Answer from the drawing. Dimensions are ordinates in mm from the lowest x, y and z of the part. A direction names the side the tool comes from. Coordinates: 2 decimals unless noted, no trailing zeros. Write each loop counter-clockwise with the first axis right and the second up, starting at its lowest first coordinate (ties: lowest second). Pieces come first, ordered by that corner, then holes.
(1) Section B-B on y = 19 is taken. Write down the section's boundary in (x, z).
(2) Section C-C on x = 40 is taken. Write down the section's boundary in (y, z), then the cut area to 3 significant figures.
(3) Section A-A on z = 28.5 is taken. Write down the section's boundary in (x, y), then the cut area to 3 significant figures.
(4) Section D-D on z = 3.5 is taken. Write down the section's boundary in (x, y).
(5) Find the intervals of material crossed by probe 1 along X at (y, z) = (90.5, 7.5); probe 2 along Y at (x, z) = (20, 24.5); probe 3 along Y at (x, z) = (23, 16), in increasing order.
(6) The mould has two halves that part along X. Classify the marked faces 4, 5 and 6: +X half, -X half, draft (parallel to the pull), parting line (faces both ways), or undercut.
(7) Given pin 1 (16 mm diameter, centred on y = 10, z = 12.5, fed in from +X); pin 2 (10 mm diameter, centred on y = 21, z = 10, fed in from -X); pin 3 (3 mm diameter, centred on x = 28.5, z = 6, fed in from +Y), each flat-ended and moving along its own axis, determine where each tip first touches the part or whether it passes through.
(8) Which of the six approach directions +Z, -Z, +X, -X, +Y, -Y give full straight-line access (tool end or side, diameter ignored) to the marked faces 1, 2 and 3?
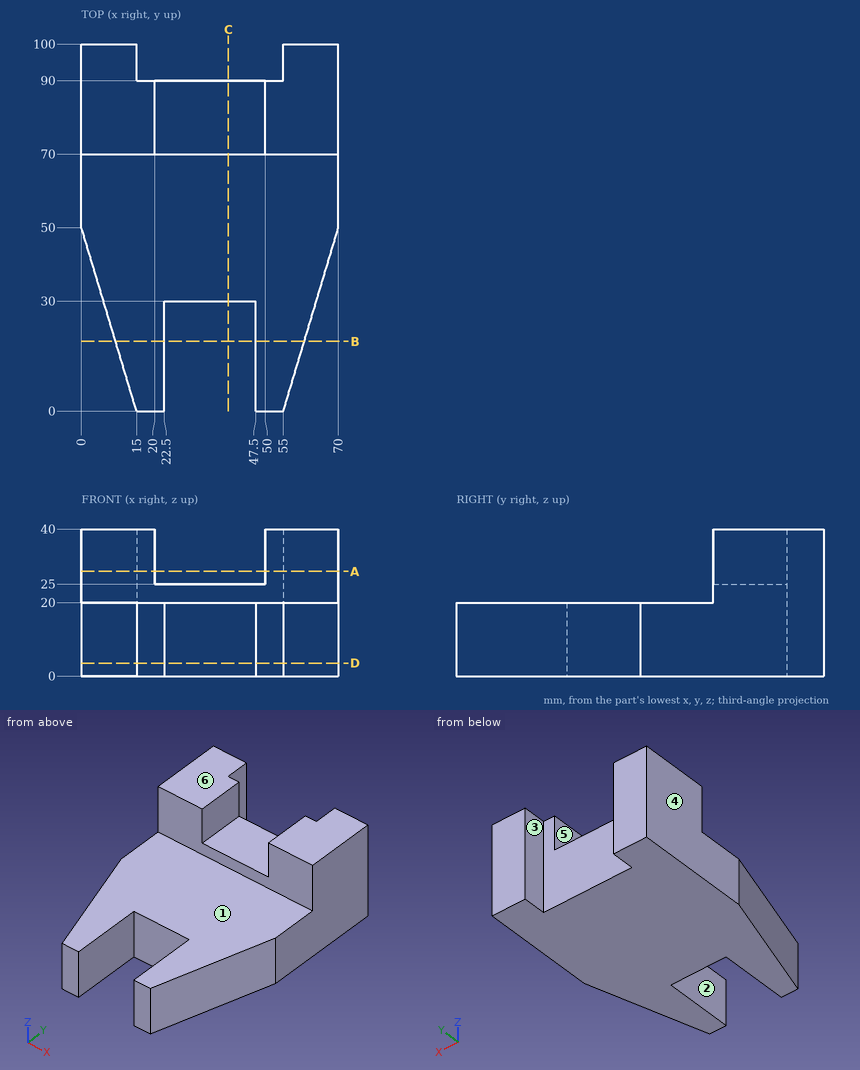
Response:
1. outline: (9.3, 0) - (22.5, 0) - (22.5, 20) - (9.3, 20) - close; (47.5, 0) - (60.7, 0) - (60.7, 20) - (47.5, 20) - close
2. outline: (30, 0) - (90, 0) - (90, 25) - (70, 25) - (70, 20) - (30, 20) - close
2. area: 1,300 mm2
3. outline: (0, 70) - (20, 70) - (20, 90) - (15, 90) - (15, 100) - (0, 100) - close; (50, 70) - (70, 70) - (70, 100) - (55, 100) - (55, 90) - (50, 90) - close
3. area: 1,100 mm2
4. outline: (0, 50) - (15, 0) - (22.5, 0) - (22.5, 30) - (47.5, 30) - (47.5, 0) - (55, 0) - (70, 50) - (70, 100) - (55, 100) - (55, 90) - (15, 90) - (15, 100) - (0, 100) - close
5. probe 1: x = 0 to 15, 55 to 70
5. probe 2: y = 70 to 90
5. probe 3: y = 30 to 90
6. face 4: -X half
6. face 5: undercut
6. face 6: draft
7. pin 1: stops at x = 60.4
7. pin 2: stops at x = 7.2
7. pin 3: stops at y = 90
8. face 1: +Z, +X, -X, -Y
8. face 2: +Z, -Z, -Y
8. face 3: +Z, -Z, +Y
